```python
from build123d import *

# Parameters (mm, degrees)
BOSS_EXTRUDE1_DEPTH = 5
SKETCH2_W           = 3
SKETCH2_H           = 12
CUT_EXTRUDE1_DEPTH  = 10
FILLET1_R           = 7
SKETCH3_R           = 1.5
CUT_EXTRUDE2_DEPTH  = 10


with BuildPart() as part:
    # Sketch1 → Boss-Extrude1 (new body)
    with BuildSketch(Plane.XY):
        with BuildLine():
            Line((13.600261452, -32.359372515), (13.600261452, -12.359372515))
            Line((13.600261452, -12.359372515), (8.600261452, -12.359372515))
            Line((8.600261452, -12.359372515), (8.600261452, 20.640627485))
            ThreePointArc((8.600261452, 20.640627485), (-5.541874172, 14.782763108), (-11.399738548, 0.640627485))
            Line((-11.399738548, 0.640627485), (-11.399738548, -27.359372515))
            Line((-11.399738548, -27.359372515), (3.600261452, -27.359372515))
            Line((3.600261452, -27.359372515), (3.600261452, -32.359372515))
            Line((3.600261452, -32.359372515), (13.600261452, -32.359372515))
        make_face()
    extrude(amount=BOSS_EXTRUDE1_DEPTH)

    # Sketch2 → Cut-Extrude1 (cut)
    with BuildSketch(Plane.XY.offset(5)):
        with Locations((-3.899738548, -21.359372515)):
            Rectangle(SKETCH2_W, SKETCH2_H)
        with BuildLine():
            Line((-6.399738548, -20.859372515), (-1.399738548, -20.859372515))
            ThreePointArc((-1.399738548, -20.859372515), (0.100261452, -22.359372515), (-1.399738548, -23.859372515))
            Line((-1.399738548, -23.859372515), (-6.399738548, -23.859372515))
            ThreePointArc((-6.399738548, -23.859372515), (-7.899738548, -22.359372515), (-6.399738548, -20.859372515))
        make_face()
    extrude(amount=-CUT_EXTRUDE1_DEPTH, mode=Mode.SUBTRACT)

    # Fillet1
    fillet1_edges = [part.edges().sort_by_distance(p)[0] for p in [
        (8.600261452, 20.640627485, 2.5),
    ]]
    fillet(fillet1_edges, radius=FILLET1_R)

    # Sketch3 → Cut-Extrude2 (cut)
    with BuildSketch(Plane.XY.offset(5)):
        with Locations((3.600261452, -17.109372515)):
            Circle(SKETCH3_R)
        with Locations((3.600261452, 12.390627485)):
            Circle(SKETCH3_R)
    extrude(amount=-CUT_EXTRUDE2_DEPTH, mode=Mode.SUBTRACT)


solid = part.part
```
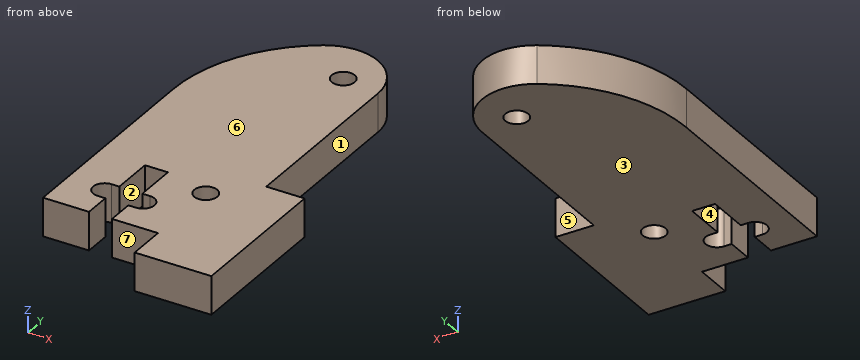
Verification items for the finished model (mm, model axes). Face numbers are marked on the shaded views. A direction names the side the tool comes from. Give positions to 0.01 mm unless a question says otherwise; leave off trailing zeros. Write each loop counter-clockwise with the first axis right and the second up, starting at its lowest first coordinate (ties: lowest second). Pieces come first, ordered by that corner, then holes. Notation, with made-up numbers: (74, 68) - (98, 68) arc R13 ccw to (98, 76) - close; hole circle Ø4 at (72.25, 12). An arc over 180 degrees is marked (long way). Put each result on its own line as item: value.
Q1. Section check D-D on y = -5.5. Record the cut outline in (x, z), and give its area (3 significant figures).
Result:
outline: (-11.4, 0) - (8.6, 0) - (8.6, 5) - (-11.4, 5) - close
area: 100 mm2
Q2. Mould release check, pull along X, two halves, no side actions. Record for the marked faces 1, 2 and 3: released by +X, released by -X, zero draft, split by the parting line, or undercut.
Result:
face 1: released by +X
face 2: undercut
face 3: zero draft
Q3. Section check A-A on y = -24.5. Record the cut outline in (x, z).
Result:
outline: (-11.4, 0) - (-5.4, 0) - (-5.4, 5) - (-11.4, 5) - close; (-2.4, 0) - (13.6, 0) - (13.6, 5) - (-2.4, 5) - close
Q4. Section check C-C on x = -9.25. Record the cut outline in (y, z).
Result:
outline: (-27.36, 0) - (9.66, 0) - (9.66, 5) - (-27.36, 5) - close
Q5. Set-up check for the marked faces 4, 5, 6 and 7: record each of +Z, -Z, +X, -X, +Y, -Y from which the full face is reachable in a straight line by a thin tool's end or side.
Result:
face 4: +Z, -Z, -Y
face 5: +Z, -Z, +X, +Y
face 6: +Z, +X, -X, +Y, -Y
face 7: +Z, -Z, -X, -Y
Q6. Depth check by flat-ended pin: P1, Ø1.5, axis at x = 1.5, z = 2, coming from the -Y side; P2, Ø8, axis at x = 9.5, y = 6.5, coming from the -Z side; P3, Ø1.1, axis at x = -2, z = 3, coming from the +Y side; P4, Ø0.9, axis at x = -4, z = 1.5, coming from the -Y side. Enter the tip coordinate at first touch or a pass-through.
Result:
P1: y = -27.36
P2: z = 0
P3: y = 17.9
P4: y = -15.36
Q7. Scan lines: probe 1 along X at (y, z) = (-19.5, 0.7); probe 2 along Y at (x, z) = (3.5, 3.15); probe 3 along Y at (x, z) = (9.75, 3). Record each from-to range of solid material in increasing order. Write a range as from..to.
Result:
probe 1: -11.4..-5.4, -2.4..13.6
probe 2: -27.36..-18.61, -15.61..10.89, 13.89..18.33
probe 3: -32.36..-12.36
Q8. Section check B-B on z = 1. Record the cut outline in (x, y).
Result:
outline: (-11.4, -27.36) - (-5.4, -27.36) - (-5.4, -23.86) - (-6.4, -23.86) arc R1.5 cw to (-6.4, -20.86) - (-5.4, -20.86) - (-5.4, -15.36) - (-2.4, -15.36) - (-2.4, -20.86) - (-1.4, -20.86) arc R1.5 cw to (-1.4, -23.86) - (-2.4, -23.86) - (-2.4, -27.36) - (3.6, -27.36) - (3.6, -32.36) - (13.6, -32.36) - (13.6, -12.36) - (8.6, -12.36) - (8.6, 11.6) arc R7 ccw to (-2.17, 17.49) arc R20 ccw to (-11.4, 0.64) - close; hole circle Ø3 at (3.6, -17.11); hole circle Ø3 at (3.6, 12.39)
